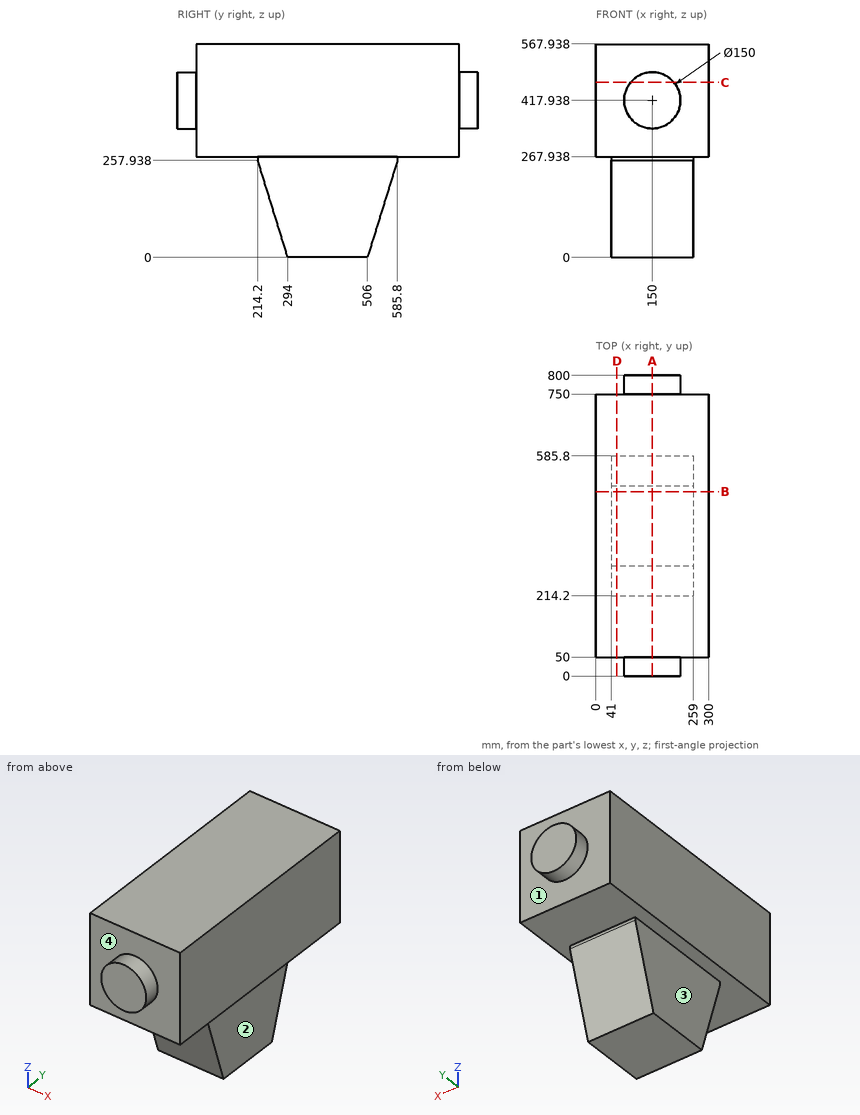
Job drawing, mm, ordinate dimensions from the low corner. One solid piece. A direction names the side the tool comes from. Round coordinates to 2 decimals unless told otherwise and drop trailing zeros. Loops run counter-clockwise (first coordinate to the right, second up) from the corner with the lowest first, then second, coordinate; pieces in that order, holes last. Notation, with made-up numbers: M 64,-15 L 69,-15 A32 ccw 69,14 Z; hole C 75,28 d9. An arc over 180 degrees is marked long. One line per question, with ' | ' between items. Start each with the question number.
Item 1: Wall check: line 1 (Z direction, x = 53, y = 65); line 2 (Y direction, x = 247, z = 263); line 3 (Y direction, x = 166, z = 525.5). Give the ranges that are in metal, low to high.
Item 2: Which spindle directions (+Z, -Z, +X, -X, +Y, -Y) get a long thin tool onto all of the face, cutting with end or side? Do the marked faces 1, 2, 3 and 4. Say none if no direction does.
Item 3: Cut at B-B, the plane y = 491. Write the cut outline in (x, z), plus the area to 3 significant figures.
Item 4: Cut at A-A, the plane x = 150. Write the cut outline in (y, z).
Item 5: Cut at C-C, the plane z = 466. Write the cut outline in (x, y).
Item 6: Pin check, flat tips, straight feed: pin 1 Ø10 at (x, z) = (221, 226.5) entering from +Y; pin 2 Ø11 at (x, z) = (190, 262) entering from -Y; pin 3 Ø12 at (y, z) = (308, 87) entering from +X. Stop position of each tip, or through.
Item 7: Cut at D-D, the plane x = 55.5. Write the cut outline in (y, z).
Responses:
1) line 1: z = 267.94 to 567.94 | line 2: y = 214.2 to 585.8 | line 3: y = 50 to 750
2) face 1: +Y | face 2: -Z, +X, +Y, -Y | face 3: -Z, -X, +Y, -Y | face 4: -Y
3) outline: M 0,267.94 L 41,267.94 L 41,0 L 259,0 L 259,267.94 L 300,267.94 L 300,567.94 L 0,567.94 Z | area: 148,000 mm²
4) outline: M 0,342.94 L 50,342.94 L 50,267.94 L 214.2,267.94 L 214.2,257.94 L 294,0 L 506,0 L 585.8,257.94 L 585.8,267.94 L 750,267.94 L 750,342.94 L 800,342.94 L 800,492.94 L 750,492.94 L 750,567.94 L 50,567.94 L 50,492.94 L 0,492.94 Z
5) outline: M 0,50 L 92.42,50 L 92.42,0 L 207.58,0 L 207.58,50 L 300,50 L 300,750 L 207.58,750 L 207.58,800 L 92.42,800 L 92.42,750 L 0,750 Z
6) pin 1: stops at y = 577.62 | pin 2: stops at y = 214.2 | pin 3: stops at x = 259
7) outline: M 50,267.94 L 214.2,267.94 L 214.2,257.94 L 294,0 L 506,0 L 585.8,257.94 L 585.8,267.94 L 750,267.94 L 750,567.94 L 50,567.94 Z
